from build123d import *

# Parameters (mm, degrees)
F0_W     = 62
F0_H     = 20
F1_DEPTH = 1
F2_W     = 62
F2_H     = 20
F2_W_2   = 60
F2_H_2   = 18
F3_DEPTH = 40
F4_R     = 5
F5_R     = 6
F6_W     = 20
F6_H     = 1
F7_DEPTH = 15
F9_DEPTH = 1
F10_R    = 7.49999


# Not quite as in the source:
# - a fillet or chamfer is up to 0.001 mm smaller than in the source, because OpenCascade refuses the exact size


with BuildPart() as f1:
    # F0 (on Top) → F1 (new body)
    with BuildSketch(Plane.XY):
        with Locations((31, 10)):
            Rectangle(F0_W, F0_H)
    extrude(amount=F1_DEPTH)

    # F2 (on face) → F3 (join)
    with BuildSketch(Plane.XY.offset(1)):
        with Locations((31, 10)):
            Rectangle(F2_W, F2_H)
        with Locations((31, 10)):
            Rectangle(F2_W_2, F2_H_2, mode=Mode.SUBTRACT)
    extrude(amount=F3_DEPTH)

    # F4
    f4_edges = [f1.edges().sort_by_distance(p)[0] for p in [
        (1, 1, 21),
        (61, 1, 21),
    ]]
    fillet(f4_edges, radius=F4_R)

    # F5
    f5_edges = [f1.edges().sort_by_distance(p)[0] for p in [
        (0, 0, 20.5),
        (62, 0, 20.5),
    ]]
    fillet(f5_edges, radius=F5_R)

    # F6 (on face) → F7 (join)
    with BuildSketch(Plane.XY.offset(41)):
        with Locations((31, 19.5)):
            Rectangle(F6_W, F6_H)
    extrude(amount=F7_DEPTH)

    # F8 (on face) → F9 (cut, through all)
    with BuildSketch(Plane.XZ.offset(-19)):
        with BuildLine():
            Line((33.4206145914, 48.625), (32.4523687548, 52.375))
            ThreePointArc((32.4523687548, 52.375), (31, 53.5), (29.5476312452, 52.375))
            Line((29.5476312452, 52.375), (28.5793854086, 48.625))
            ThreePointArc((28.5793854086, 48.625), (31, 45.5), (33.4206145914, 48.625))
        make_face()
    extrude(amount=-F9_DEPTH, mode=Mode.SUBTRACT)

    # F10 (radius 7.5 in the source; OpenCascade refuses exactly that, so slightly less here)
    f10_edges = [f1.edges().sort_by_distance(p)[0] for p in [
        (21, 19.5, 56),
        (41, 19.5, 56),
        (41, 19.5, 41),
        (21, 19.5, 41),
    ]]
    fillet(f10_edges, radius=F10_R)


solid = f1.part
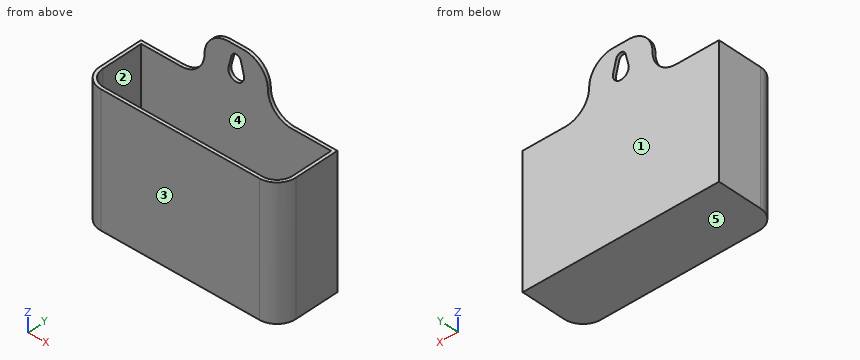
Model file for the job. Use its own axes, mm. Face numbers are marked on the shaded views. A direction names the side the tool comes from. Give positions to 0.01 mm unless a question says otherwise; leave off trailing zeros. Order: outer loops, then holes, each group sorted by start corner. A loop starts at its lowest first (then second) coordinate and runs counter-clockwise, first axis right, second up. Notation, with made-up numbers: (-13, 59.25) - (-2, 59.25) arc R16 ccw to (-2, 82.25) - close; hole circle Ø10 at (80, 32). An arc over 180 degrees is marked (long way). Write item = value, one per line. Start each with the question number.
1. Cut at B-B, the plane z = 32. List the corners of the cut face in (x, y).
2. Cut at D-D, the plane x = 11. List the corners of the cut face in (y, z), and give its area (3 significant figures).
3. Two-plate mould, pull along Y, no slides. Class the marked faces 3, 4 and 5: pulls with the +Y half, pulls with the -Y half, needs draft (parallel to the pull), parting line crosses it, or undercut.
4. Cut at C-C, the plane y = 15.25. List the corners of the cut face in (x, z), and give its area (3 significant figures).
5. Probe line 1 along X through (y, z) = (19.8, 48); line 2 along X through (y, z) = (10.5, 10); line 3 along Y through (x, z) = (49, 36.5). List the from-to ranges inside material, lowest first.
6. Cut at A-A, the plane x = 31. List the corners of the cut face in (y, z).
7. Which spindle directions (+Z, -Z, +X, -X, +Y, -Y) get a long thin tool onto all of the face, cutting with end or side? Do the marked faces 1 and 2. Say none if no direction does.
8. Drop flat-ended pins along their axis: P1, Ø3, axis at x = 31, z = 48, coming from the -Y side; P2, Ø8, axis at x = 42.5, y = 8.5, coming from the +Z side; P3, Ø12, axis at x = 44, y = 5, coming from the +Z side. Give the stop position or say it passes through.
Taken from the geometry:
q1.outline = (0, 6) arc R6 ccw to (6, 0) - (56, 0) arc R6 ccw to (62, 6) - (62, 20) - (0, 20) - close; hole (1, 6) arc R5 ccw to (6, 1) - (56, 1) arc R5 ccw to (61, 6) - (61, 19) - (1, 19) - close
q2.outline = (0, 0) - (20, 0) - (20, 41) - (19, 41) - (19, 1) - (1, 1) - (1, 41) - (0, 41) - close
q2.area = 100 mm²
q3.face_3 = pulls with the -Y half
q3.face_4 = undercut
q3.face_5 = needs draft
q4.outline = (0, 0) - (62, 0) - (62, 41) - (61, 41) - (61, 1) - (1, 1) - (1, 41) - (0, 41) - close
q4.area = 142 mm²
q5.line_1 = 20.98 to 28.5, 33.5 to 41.02
q5.line_2 = 0 to 1, 61 to 62
q5.line_3 = 0 to 1, 19 to 20
q6.outline = (0, 0) - (20, 0) - (20, 45.5) - (19, 45.5) - (19, 1) - (1, 1) - (1, 41) - (0, 41) - close; (19, 53.5) - (20, 53.5) - (20, 56) - (19, 56) - close
q7.face_1 = +Z, -Z, +X, -X, +Y
q7.face_2 = +Z
q8.P1 = through
q8.P2 = 1
q8.P3 = 41
